Can you work these out from the drawing? Everything is in mm from the part's minimum corner. A direction names the side the tool comes from. Round coordinates to 2 decimals unless told otherwise and drop trailing zeros. Write each loop counter-clockwise with the first axis right and the second up, starting at its lowest first coordinate (ties: lowest second). Pieces come first, ordered by that corner, then holes. Notation, with made-up numbers: (70, 19.25) -> (76, 19.25) arc R20 ccw to (76, 48.25) -> close; hole circle Ø11 at (88, 1.5). An arc over 180 degrees is marked (long way). Put each result on its own line as item: value. Start each with the question number.
1. Suppose I cut it at A-A (z = 3.5). Please give me the cut outline in (x, y), then the cut area to 3 significant figures.
2. Suppose I cut it at D-D (z = 9.25). Please give me the cut outline in (x, y).
3. Which directions (+Z, -Z, +X, -X, +Y, -Y) give clear straight access to the entire face, cutting with the end or side of a thin tool? Please do the marked faces 5 and 6.
4. Suppose I cut it at B-B (y = 10.5). Please give me the cut outline in (x, z), then the cut area to 3 significant figures.
5. I need wall thicknesses on probe 1 along X at (y, z) = (13, 1.75); probe 2 along Z at (x, y) = (68, 5.25). Which ranges of each line are inside material? Lowest first, please. Write a range as from..to.
6. For pin 1 (3 mm diameter, centred on x = 60.5, y = 7.5, fed in from +Z); pin 2 (1.5 mm diameter, centred on x = 88, y = 4, fed in from -Z); pin 3 (1.5 mm diameter, centred on y = 3, z = 10.5, fed in from -X); pin 4 (1.5 mm diameter, centred on x = 105.5, z = 14.5, fed in from -Y), each with a flat end and sliding along its axis, tell me the tip position at first contact or that it passes through.
7. We'd pull the mould along X, two halves only. Please class the marked faces 1, 2, 3 and 4: +X half, -X half, draft (parallel to the pull), parting line (faces both ways), or undercut.
8. Suppose I cut it at C-C (x = 10). Please give me the cut outline in (y, z), then the cut area to 3 significant figures.
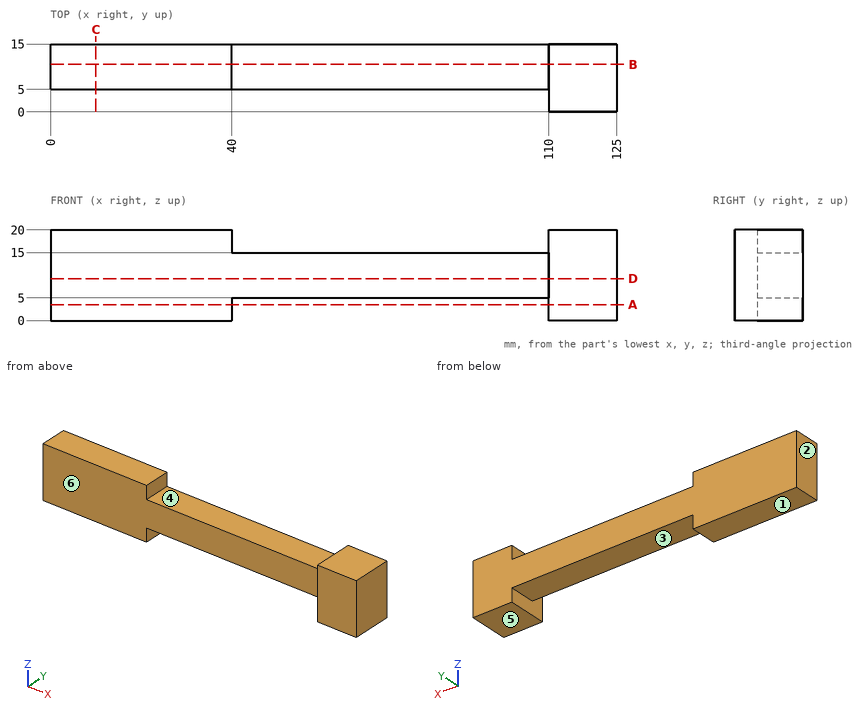
Verdict:
1. outline: (0, 5) -> (40, 5) -> (40, 15) -> (0, 15) -> close; (110, 0) -> (125, 0) -> (125, 15) -> (110, 15) -> close
1. area: 625 mm^2
2. outline: (0, 5) -> (110, 5) -> (110, 0) -> (125, 0) -> (125, 15) -> (0, 15) -> close
3. face 5: -Z, +X, -X, +Y, -Y
3. face 6: +Z, -Z, -X, -Y
4. outline: (0, 0) -> (40, 0) -> (40, 5) -> (110, 5) -> (110, 0) -> (125, 0) -> (125, 20) -> (110, 20) -> (110, 15) -> (40, 15) -> (40, 20) -> (0, 20) -> close
4. area: 1,800 mm^2
5. probe 1: x = 0..40, 110..125
5. probe 2: z = 5..15
6. pin 1: stops at z = 15
6. pin 2: passes through
6. pin 3: stops at x = 110
6. pin 4: stops at y = 5
7. face 1: draft
7. face 2: -X half
7. face 3: undercut
7. face 4: undercut
8. outline: (5, 0) -> (15, 0) -> (15, 20) -> (5, 20) -> close
8. area: 200 mm^2
